Read the model definition and answer for the solid it produces. Units are mm, in the model's axes. Face numbers are marked on the shaded views. A direction names the side the tool comes from. Give positions to 0.01 mm unless a question says otherwise; leave off trailing zeros. Order: outer loops, then holes, each group sorted by start corner. A loop starts at its lowest first (then second) coordinate and runs counter-clockwise, first axis right, second up. Notation, with made-up numbers: (82.5, 79.25) -> (140.5, 79.25) arc R35 ccw to (140.5, 115.25) -> close; hole circle Ø10 at (87.25, 65). An arc over 180 degrees is marked (long way). One line per question, with ' | ' between items. Start each with the question number.
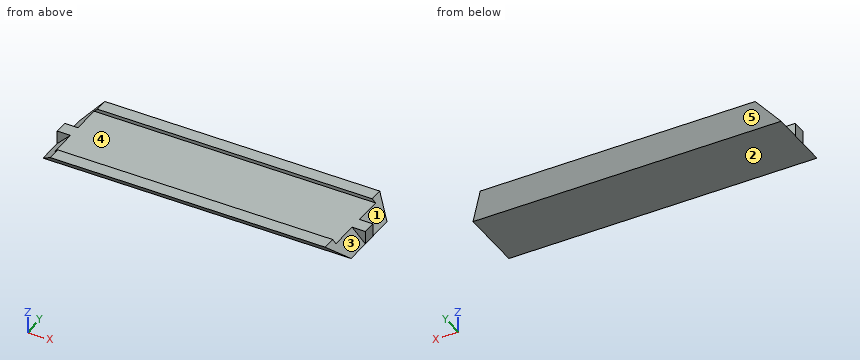
Autodesk Inventor part; units mm, degrees
ref_plane "Work Plane1" through (0, 0, -23.368) normal (0, 0, -1) x (-1, 0, 0)
ref_plane "YZ Plane" through (0, 0, 0) normal (1, 0, 0) x (0, 1, 0)
ref_plane "XZ Plane" through (0, 0, 0) normal (0, 1, 0) x (-1, 0, 0)
sketch "Sketch1" plane through (0, 0, 0) normal (0, 0, 1) x (1, 0, 0)
  line L0 (0, 0) -> (33.274, 0)
  line L1 (33.274, 0) -> (33.274, 13.462)
  line L2 (33.274, 13.462) -> (0, 13.462)
  line L3 (0, 13.462) -> (0, 0)
  line L4 (-2.54, 16.002) -> (35.814, 16.002)
  line L5 (35.814, 16.002) -> (35.814, -2.54)
  line L6 (35.814, -2.54) -> (-2.54, -2.54)
  line L7 (-2.54, -2.54) -> (-2.54, 16.002)
  dimension "d0" = 33.274
  dimension "d1" = 13.462
  dimension "d2" = 2.54
extrude "Extrusion1" add sketch "Sketch1" against normal blind 13.208
sketch "Sketch3" plane through (0, 0, 0) normal (0, 0, 1) x (1, 0, 0)
  line L0 (14.986, 16.002) -> (14.986, 13.462)
  line L1 (0, 13.462) -> (33.274, 13.462)
  line L2 (35.814, 16.002) -> (-2.54, 16.002)
  line L3 (-2.54, 16.002) -> (-2.54, -2.54)
  line L4 (18.288, 16.002) -> (18.288, 13.462)
  line L5 (35.814, -2.54) -> (35.814, 16.002)
  line L6 (14.986, 16.002) -> (18.288, 16.002)
  line L7 (18.288, 13.462) -> (14.986, 13.462)
  line L8 (33.274, 13.462) -> (33.274, 0)
  line L9 (0, 0) -> (0, 13.462)
  dimension "d5" = 0
  dimension "d6" = 0
  dimension "d7" = 14.986
  dimension "d8" = 14.986
extrude "Extrusion2" cut sketch "Sketch3" against normal blind 7.62
sketch "Sketch4" plane through (0, 0, 0) normal (0, 1, 0) x (-1, 0, 0)
  line L0 (10.287, -23.368) -> (-43.561, -23.368)
  line L1 (-43.561, -23.368) -> (-43.561, -94.234)
  line L2 (-43.561, -94.234) -> (10.287, -94.234)
  line L3 (10.287, -94.234) -> (10.287, -23.368)
  circle A0 centre (-41.529, -25.4) radius 1.016
  circle A1 centre (8.255, -25.4) radius 1.016
  circle A2 centre (8.255, -92.202) radius 1.016
  circle A3 centre (-41.529, -92.202) radius 1.016
  line L4 (-33.274, -13.208) -> (0, -13.208)
  line L5 (-16.637, -13.208) -> (-16.637, -16.4825)
  point P0 (0, 0)
  dimension "d11" = 53.848
  dimension "d12" = 70.866
  dimension "d14" = 2.032
  dimension "d15" = 2.032
  dimension "d16" = 2.032
  dimension "d17" = 2.032
  dimension "d18" = 2.032
  dimension "d19" = 2.032
  dimension "d20" = 2.032
  dimension "d21" = 2.032
  dimension "d22" = 2.032
  dimension "d23" = 2.032
  dimension "d24" = 2.032
  dimension "d25" = 2.032
  dimension "d26" = 26.924
  dimension "d27" = 10.16
ref_plane "Work Plane1" through (0, 0, -23.368) normal (0, 0, -1) x (-1, 0, 0)
sketch "Sketch5" plane through (0, 0, -23.368) normal (0, 0, -1) x (-1, 0, 0)
  line L0 (10.287, 0) -> (-43.561, 0)
  line L1 (-43.561, 0) -> (10.287, 0)
  line L2 (10.287, 13.462) -> (10.287, 0)
  line L3 (10.287, 0) -> (-43.561, 0)
  line L4 (12.827, -2.54) -> (-46.101, -2.54)
  line L5 (-46.101, -2.54) -> (-46.101, 16.002)
  line L6 (-46.101, -2.54) -> (12.827, -2.54)
  line L7 (12.827, -2.54) -> (12.827, 16.002)
  line L8 (12.827, 16.002) -> (-46.101, 16.002)
  line L9 (-46.101, 16.002) -> (-46.101, -2.54)
  line L10 (10.287, 0) -> (-43.561, 0)
  line L11 (-43.561, 0) -> (-43.561, 13.462)
  line L12 (-43.561, 13.462) -> (10.287, 13.462)
  line L13 (10.287, 13.462) -> (10.287, 0)
  point P0 (0, 0)
sketch "Sketch6" plane through (0, 0, -13.208) normal (0, 0, -1) x (-1, 0, 0)
  line L0 (-35.814, -2.54) -> (2.54, -2.54)
  line L1 (2.54, -2.54) -> (2.54, 16.002)
  line L2 (2.54, 16.002) -> (-35.814, 16.002)
  line L3 (-35.814, 16.002) -> (-35.814, -2.54)
  line L4 (0, 13.462) -> (0, 0)
  line L5 (0, 0) -> (-33.274, 0)
  line L6 (-33.274, 0) -> (-33.274, 13.462)
  line L7 (-33.274, 13.462) -> (0, 13.462)
extrude "Extrusion3" add sketch "Sketch5" along normal blind 73.406
sketch "Sketch7" plane through (0, 0, -23.368) normal (0, 0, 1) x (1, 0, 0)
  line L0 (46.101, 16.002) -> (46.101, -2.54)
  line L1 (-12.827, 16.002) -> (46.101, 16.002)
  line L2 (-12.827, -2.54) -> (-12.827, 16.002)
  line L3 (46.101, -2.54) -> (-12.827, -2.54)
  line L4 (43.561, 13.462) -> (-10.287, 13.462)
  line L5 (43.561, 0) -> (43.561, 13.462)
  line L6 (-10.287, 0) -> (43.561, 0)
  line L7 (-10.287, 13.462) -> (-10.287, 0)
  point P0 (0, 0)
sketch "Sketch8" plane through (0, 0, -23.368) normal (0, 0, 1) x (1, 0, 0)
  point P0 (0, 0)
sketch "Sketch9" plane through (0, 0, 0) normal (0, 1, 0) x (-1, 0, 0)
  line L0 (2.54, -13.208) -> (-35.814, -13.208)
  line L1 (12.827, -23.368) -> (2.54, -13.208)
  line L2 (2.54, -13.208) -> (-35.814, -13.208)
  line L3 (-45.8486, -23.368) -> (12.827, -23.368)
  line L4 (-35.814, 0) -> (-35.814, -13.208)
  line L5 (-46.101, -23.368) -> (12.827, -23.368)
  line L6 (-35.814, -13.208) -> (-46.101, -23.368)
  line L7 (-46.101, -23.368) -> (12.827, -23.368)
  point P0 (0, 0)
extrude "Extrusion5" add sketch "Sketch9" against normal blind 2.54
sketch "Sketch11" plane through (0, 0, 0) normal (0, 1, 0) x (1, 0, 0)
  line L0 (33.274, 0) -> (0, 0)
  line L1 (33.274, 0) -> (33.274, 13.208)
  line L2 (35.814, 13.208) -> (33.274, 13.208)
  line L3 (35.814, 13.208) -> (46.101, 23.368)
  line L4 (43.561, 23.368) -> (46.101, 23.368)
  line L5 (43.561, 23.368) -> (43.561, 96.774)
  line L6 (-10.287, 96.774) -> (43.561, 96.774)
  line L7 (-10.287, 23.368) -> (-10.287, 96.774)
  line L8 (-12.827, 23.368) -> (-10.287, 23.368)
  line L9 (-12.827, 23.368) -> (-2.54, 13.208)
  line L10 (0, 13.208) -> (-2.54, 13.208)
  line L11 (0, 0) -> (0, 13.208)
  line L12 (-12.827, 23.368) -> (-2.54, 13.208)
  line L13 (-11.0421, 25.1752) -> (0, 14.2694)
  line L14 (0, 0) -> (0, 13.208)
  line L15 (0, 13.208) -> (0, 14.2694)
  line L16 (-10.287, 23.368) -> (-10.287, 96.774)
  line L17 (-10.287, 24.4294) -> (-10.287, 23.368)
  line L18 (-12.827, 23.368) -> (-10.287, 23.368)
  line L19 (-10.287, 23.368) -> (-12.827, 23.368)
  line L20 (-2.54, 0) -> (-2.54, 13.208)
  line L21 (-12.827, 23.368) -> (-2.54, 13.208)
  line L22 (-2.54, 13.208) -> (0, 13.208)
  line L23 (16.637, 13.208) -> (16.637, 17.9384)
  line L24 (46.101, 23.368) -> (43.561, 23.368)
  line L25 (46.101, 23.368) -> (35.814, 13.208)
  line L26 (44.3161, 25.1752) -> (33.274, 14.2694)
  line L27 (33.274, 13.208) -> (33.274, 14.2694)
  line L28 (43.561, 24.4294) -> (43.561, 23.368)
  line L29 (35.814, 13.208) -> (33.274, 13.208)
  point P0 (43.561, 24.4294)
  dimension "d40" = 2.54
extrude "Extrusion7" add sketch "Sketch11" along normal up to surface (13.462 mm away) contours L27 L26 L5 L4 L3 L2 | L10 L9 L8 L7 L13 L15
sketch "Sketch12" plane through (-12.827, 13.462, -23.368) normal (0, 1, 0) x (1, 0, 0)
  line L0 (58.928, 0) -> (55.3134, 0)
  line L1 (55.3134, 0) -> (46.101, -9.0986)
  line L2 (46.101, -9.0986) -> (46.101, -10.16)
  line L3 (48.641, -10.16) -> (46.101, -10.16)
  line L4 (48.641, -10.16) -> (58.928, 0)
  line L5 (3.6146, 0) -> (0, 0)
  line L6 (0, 0) -> (10.287, -10.16)
  line L7 (12.827, -10.16) -> (10.287, -10.16)
  line L8 (12.827, -10.16) -> (12.827, -9.0986)
  line L9 (12.827, -9.0986) -> (3.6146, 0)
  line L10 (12.827, -23.368) -> (12.827, -10.16)
  line L11 (12.827, -10.16) -> (46.101, -10.16)
  line L12 (55.3134, 0) -> (3.6146, 0)
  line L13 (55.3134, 0) -> (3.6146, 0)
extrude "Extrusion8" add sketch "Sketch12" along normal blind 2.54
sketch "Sketch13" plane through (0, 0, 0) normal (0, 1, 0) x (1, 0, 0)
  line L0 (43.561, 94.234) -> (-10.287, 94.234)
  line L1 (46.101, 96.774) -> (-12.827, 96.774)
  line L2 (-10.287, 94.234) -> (43.561, 94.234)
  line L3 (43.561, 94.234) -> (43.561, 96.774)
  line L4 (43.561, 96.774) -> (-10.287, 96.774)
  line L5 (-10.287, 96.774) -> (-10.287, 94.234)
  point P0 (0, 0)
  point P1 (-10.287, 96.774)
extrude "Extrusion9" add sketch "Sketch13" along normal up to next
chamfer "Chamfer1" distance 3.175 angle 45 14 edges at (-12.827, 16.002, -60.071) (46.101, 16.002, -60.071) (46.101, -2.54, -60.071) (-12.827, -2.54, -60.071) (16.637, 16.002, -96.774) (16.637, -2.54, -96.774) (40.9575, 16.002, -18.288) (40.9575, -2.54, -18.288) (-7.6835, 16.002, -18.288) (-7.6835, -2.54, -18.288) (35.814, 16.002, -6.604) (35.814, -2.54, -6.604) (-2.54, 16.002, -6.604) (-2.54, -2.54, -6.604)
sketch "Sketch15" plane through (14.986, 16.002, -7.62) normal (0, 1, 0) x (1, 0, 0)
  line L0 (17.653, 6.9147) -> (17.653, -7.62)
  line L1 (17.653, -7.62) -> (20.828, -7.62)
  line L2 (20.828, -7.62) -> (20.828, 5.588)
  line L3 (20.828, 5.588) -> (17.653, 6.9147)
  line L4 (17.653, 6.9147) -> (17.653, -7.62)
  line L5 (27.94, 17.0747) -> (17.653, 6.9147)
  line L6 (27.94, 85.979) -> (27.94, 17.0747)
  line L7 (-24.638, 85.979) -> (27.94, 85.979)
  line L8 (-24.638, 17.0747) -> (-24.638, 85.979)
  line L9 (-14.351, 6.9147) -> (-24.638, 17.0747)
  line L10 (-14.351, -7.62) -> (-14.351, 6.9147)
  line L11 (0, -7.62) -> (-14.351, -7.62)
  line L12 (0, -7.62) -> (0, 0)
  line L13 (0, 0) -> (3.302, 0)
  line L14 (3.302, 0) -> (3.302, -7.62)
  line L15 (17.653, -7.62) -> (3.302, -7.62)
  line L16 (-17.526, 5.588) -> (-17.526, -7.62)
  line L17 (-17.526, -7.62) -> (-14.351, -7.62)
  line L18 (-14.351, -7.62) -> (-14.351, 6.9147)
  line L19 (-14.351, 6.9147) -> (-17.526, 5.588)
  line L20 (-14.351, 6.9147) -> (-24.638, 17.0747)
  line L21 (-24.638, 17.0747) -> (-27.813, 15.748)
  line L22 (-27.813, 15.748) -> (-17.526, 5.588)
  line L23 (-14.351, 6.9147) -> (-17.526, 5.588)
  line L24 (-27.813, 89.154) -> (-27.813, 15.748)
  line L25 (-24.638, 17.0747) -> (-27.813, 15.748)
  line L26 (-24.638, 17.0747) -> (-24.638, 85.979)
  line L27 (-24.638, 85.979) -> (-27.813, 89.154)
  line L28 (31.115, 15.748) -> (31.115, 89.154)
  line L29 (-25.273, 16.8094) -> (-25.273, 86.614)
  line L30 (-25.273, 16.8094) -> (-14.986, 6.6494)
  line L31 (-14.986, -7.62) -> (-14.986, 6.6494)
  line L32 (18.288, -7.62) -> (-14.986, -7.62)
  line L33 (18.288, -7.62) -> (18.288, 6.6494)
  line L34 (18.288, 6.6494) -> (28.575, 16.8094)
  line L35 (28.575, 16.8094) -> (28.575, 86.614)
  line L36 (20.828, 5.588) -> (31.115, 15.748)
  line L37 (20.828, 5.588) -> (31.115, 15.748)
  line L38 (27.94, 17.0747) -> (31.115, 15.748)
  line L39 (27.94, 17.0747) -> (17.653, 6.9147)
  line L40 (20.828, 5.588) -> (17.653, 6.9147)
  line L41 (31.115, 15.748) -> (31.115, 89.154)
  line L42 (31.115, 89.154) -> (27.94, 85.979)
  line L43 (27.94, 85.979) -> (27.94, 17.0747)
  line L44 (27.94, 17.0747) -> (31.115, 15.748)
extrude "Extrusion10" cut sketch "Sketch15" against normal through all
sketch "Sketch16" plane through (-10.287, 0, -94.234) normal (0, 0, 1) x (1, 0, 0)
  line L0 (0, 0) -> (0.635, 0)
  line L1 (0, 0) -> (0, 13.462)
  line L2 (0.635, 13.462) -> (0, 13.462)
  line L3 (0.635, 16.002) -> (0.635, 13.462)
  line L4 (0.635, 16.002) -> (-2.54, 12.827)
  line L5 (-2.54, 0.635) -> (-2.54, 12.827)
  line L6 (-2.54, 0.635) -> (0.635, -2.54)
  line L7 (0.635, 0) -> (0.635, -2.54)
  line L8 (53.213, 0) -> (53.848, 0)
  line L9 (53.213, 0) -> (53.213, -2.54)
  line L10 (53.213, -2.54) -> (56.388, 0.635)
  line L11 (56.388, 12.827) -> (56.388, 0.635)
  line L12 (56.388, 12.827) -> (53.213, 16.002)
  line L13 (53.213, 16.002) -> (53.213, 13.462)
  line L14 (53.848, 13.462) -> (53.213, 13.462)
  line L15 (53.848, 13.462) -> (53.848, 0)
  line L16 (0, 0) -> (0, 13.462)
  line L17 (-2.54, 0.635) -> (-2.54, 12.827)
  line L18 (0, 8.001) -> (-2.54, 8.001)
  line L19 (0, 5.461) -> (-2.54, 5.461)
  line L20 (-2.54, 8.001) -> (0, 8.001)
  line L21 (0, 8.001) -> (0, 5.461)
  line L22 (0, 5.461) -> (-2.54, 5.461)
  line L23 (-2.54, 5.461) -> (-2.54, 8.001)
  line L24 (53.848, 13.462) -> (53.848, 0)
  line L25 (56.388, 12.827) -> (56.388, 0.635)
  line L26 (53.848, 5.461) -> (56.388, 5.461)
  line L27 (56.388, 5.461) -> (56.388, 8.001)
  line L28 (56.388, 8.001) -> (53.848, 8.001)
  line L29 (53.848, 8.001) -> (53.848, 5.461)
  point P0 (10.287, 0)
  point P1 (-2.54, 5.461)
  point P2 (0, 5.461)
  point P3 (0, 8.001)
  point P4 (-2.54, 8.001)
extrude "Extrusion11" add sketch "Sketch16" against normal up to surface (2.54 mm away) contours L19 L5 L18 L1 | L15 L28 L11 L26
properties part number "Cap"
Q1. Find the intervals of material crossed by line 1 (Z direction, x = -3, y = 11); line 2 (Y direction, x = 24, z = -93.75); line 3 (Y direction, x = 5, z = -94.7), in increasing order.
Q2. Which of the six approach directions +Z, -Z, +X, -X, +Y, -Y give full straight-line access (tool end or side, diameter ignored) to the marked faces 1, 2, 3, 4 and 5?
Q3. Given P1, Ø6, axis at x = 16.5, y = 0.5, coming from the +Z side; P2, Ø1, axis at x = 6, z = -95.5, coming from the -Y side; P3, Ø1.5, axis at x = 32, z = -96, coming from the +Y side; P4, Ø1.3, axis at x = -11, z = -96, coming from the +Y side, each flat-ended and moving along its own axis, determine where each tip first touches the part or whether it passes through.
Q4. A cutting plane is placed at C-C, the plane y = 11.75. Determine the outline of the cut face in (x, z), then the cut area to 3 significant figures.
Q5. A cutting plane is placed at A-A, the plane x = 17. Determine the outline of the cut face in (y, z) (3 decimals), then the cut area to 3 significant figures.
Q6. A cutting plane is placed at B-B, the plane z = -96.05. Determine the outline of the cut face in (x, y), then the cut area to 3 significant figures.
Geometry results:
1) line 1: -96.77 to -94.23 | line 2: -2.39 to 0, 13.46 to 15.85 | line 3: -1.44 to 14.9
2) face 1: +Z, +X, +Y | face 2: -Z, +X, -X, +Y, -Y | face 3: +Z, +X, -Y | face 4: +Z, +X, -X | face 5: -Z, +X, -X, +Y
3) P1: z = -93.6 | P2: y = -1.14 | P3: y = 14.35 | P4: y = 14.25
4) outline: (-12.83, -96.77) -> (46.1, -96.77) -> (43.56, -94.23) -> (-10.29, -94.23) -> close | area: 143 mm²
5) outline: (-2.54, -93.599) -> (0.635, -96.774) -> (12.827, -96.774) -> (16.002, -93.599) -> (13.462, -93.599) -> (13.462, -94.234) -> (0, -94.234) -> (0, -93.599) -> close | area: 40.2 mm²
6) outline: (-12.83, 5.46) -> (-12.1, 5.46) -> (-12.1, -0.09) -> (45.38, -0.09) -> (45.38, 5.46) -> (46.1, 5.46) -> (46.1, 8) -> (45.38, 8) -> (45.38, 13.55) -> (-12.1, 13.55) -> (-12.1, 8) -> (-12.83, 8) -> close | area: 788 mm²
